Source: CAD feature listing. Evaluate the final solid. Frame: model axes, mm. Face numbers are marked on the shaded views. A direction names the side the tool comes from. Round coordinates to 2 decimals unless told otherwise and drop trailing zeros. Write each loop counter-clockwise with the first axis right and the second up, starting at its lowest first coordinate (ties: lowest second). Pieces come first, ordered by that corner, then holes. Notation, with made-up numbers: M 34.5,50 L 89.5,50 A22 cw 89.5,89 Z; hole C 40.5,-25.5 d4. An arc over 180 degrees is marked long. Answer in a Markdown table with one row per item. Add a question column.
Item 1: Contact query for a flat-ended pin moving along its axis: pin 1 (2 mm diameter, centred on y = 6, z = -5, fed in from +X). Output: stop coordinate, or through.
Item 2: Material intervals for probe 1 along X at (y, z) = (1.75, 0.75); probe 2 along X at (y, z) = (4.75, -3); probe 3 along Z at (x, y) = (3.75, 2), sorted ascending.
Item 3: Set-up query: the marked faces 4, 5 and 6. Return all of +Z, -Z, +X, -X, +Y, -Y with unobstructed straight access to the full face (end or side cutting, diameter ignored); none if empty.
Item 4: Cut plane A-A on y = 2. Return loops of the section in (x, z), and give its area (3 significant figures).
Item 5: Mould query, pull axis X, two halves, no side actions, for the marked faces 1, 2 and 3. Classes: released by +X, released by -X, zero draft, split by the parting line, or undercut.
from build123d import *

# Parameters (mm, degrees)
SKETCH1_W                        = 20
SKETCH1_H                        = 20
BOSS_EXTRUDE1_DEPTH              = 7
F_10_0MM_CLEARANCE_DOWEL_HOLE1_D = 10
CUT_EXTRUDE1_DEPTH               = 16.779733838
FILLET1_R                        = 1


with BuildPart() as part:
    # Sketch1 → Boss-Extrude1 (new body)
    with BuildSketch(Plane(origin=(0, 0, 0), x_dir=(1, 0, 0), z_dir=(0, 1, 0))):
        Rectangle(SKETCH1_W, SKETCH1_H)
    extrude(amount=BOSS_EXTRUDE1_DEPTH)

    # Ø10.0mm Clearance Dowel Hole1 (through all)
    with Locations(Plane(origin=(0, 7, 0), x_dir=(1, 0, 0), z_dir=(0, 1, 0))):
        with Locations((0, 0)):
            Hole(F_10_0MM_CLEARANCE_DOWEL_HOLE1_D / 2)

    # Sketch6 → Cut-Extrude1 (cut, through all)
    with BuildSketch(Plane(origin=(0, 7, 0), x_dir=(1, 0, 0), z_dir=(0, 1, 0))):
        Polygon((-10, 10), (-10, 0.058741053), (-4.949128756, 8.689624564), (5.050871244, 8.630883511), (10, -0.058741053), (10, 10), align=None)
        Polygon((4.949128756, -8.689624564), (-5.050871244, -8.630883511), (-10, 0.058741053), (-10, -10), (10, -10), (10, -0.058741053), align=None)
    extrude(amount=-CUT_EXTRUDE1_DEPTH, mode=Mode.SUBTRACT)

    # Fillet1
    fillet1_edges = [part.edges().sort_by_distance(p)[0] for p in [
        (5, 7, 0),
        (5, 0, 0),
        (-7.474564378, 7, -4.374182809),
        (7.525435622, 7, -4.286071229),
        (0.050871244, 7, -8.660254038),
        (-7.474564378, 0, -4.374182809),
        (7.525435622, 0, -4.286071229),
        (0.050871244, 0, -8.660254038),
        (-7.525435622, 7, 4.286071229),
        (-0.050871244, 7, 8.660254038),
        (7.474564378, 7, 4.374182809),
        (-7.525435622, 0, 4.286071229),
        (-0.050871244, 0, 8.660254038),
        (7.474564378, 0, 4.374182809),
    ]]
    fillet(fillet1_edges, radius=FILLET1_R)


solid = part.part
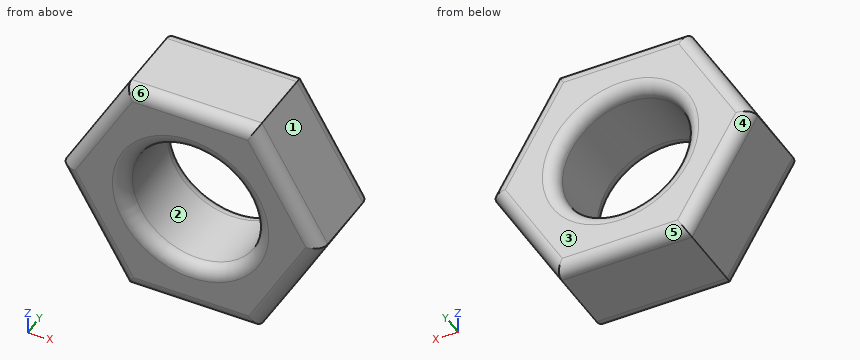
Results below:
| question | item | result |
|---|---|---|
| 1 | pin 1 | x = 7.69 |
| 2 | probe 1 | -9.54 to -4.94, 4.94 to 9.6 |
| 2 | probe 2 | -8.28 to -4, 4 to 8.26 |
| 2 | probe 3 | -8.64 to -3.31, 3.31 to 8.68 |
| 3 | face 4 | -Z, -X, +Y |
| 3 | face 5 | -Z, +X, +Y |
| 3 | face 6 | +Z, -X, -Y |
| 4 | outline | M -10,-0.06 L -4.95,-8.69 L 5.05,-8.63 L 10,0.06 L 4.95,8.69 L -5.05,8.63 Z; hole C 0,0 d10 |
| 4 | area | 181 mm2 |
| 5 | face 1 | released by +X |
| 5 | face 2 | undercut |
| 5 | face 3 | zero draft |
